```python
from build123d import *

# Parameters (mm, degrees)
SALIENTE_EXTRUIR1_DEPTH = 3


with BuildPart() as part:
    # Croquis1 → Saliente-Extruir1 (new body)
    with BuildSketch(Plane.XY):
        Polygon((-32.5, 0), (24.75, 0), (24.75, 3), (32.5, 3), (32.5, 0), (32.5, -158), (32.5, -161), (24.75, -161), (24.75, -158), (-32.5, -158), align=None)
        Polygon((-13.175, -7.03), (-25.475, -19.33), (-25.475, -7.03), align=None, mode=Mode.SUBTRACT)
        Polygon((13.175, -7.03), (25.475, -7.03), (25.475, -19.33), align=None, mode=Mode.SUBTRACT)
        Polygon((13.175, -79), (25.475, -66.7), (25.475, -91.3), align=None, mode=Mode.SUBTRACT)
        Polygon((13.175, -150.97), (25.475, -138.67), (25.475, -150.97), align=None, mode=Mode.SUBTRACT)
        Polygon((-13.175, -79), (-25.475, -66.7), (-25.475, -91.3), align=None, mode=Mode.SUBTRACT)
        Polygon((13.175, -43.015), (25.475, -55.315), (25.475, -30.715), align=None, mode=Mode.SUBTRACT)
        Polygon((-13.175, -43.015), (-25.475, -30.715), (-25.475, -55.315), align=None, mode=Mode.SUBTRACT)
        Polygon((0, -48.7075), (-12.3, -61.0075), (0, -73.3075), (12.3, -61.0075), align=None, mode=Mode.SUBTRACT)
        Polygon((0, -12.7225), (12.3, -25.0225), (0, -37.3225), (-12.3, -25.0225), align=None, mode=Mode.SUBTRACT)
        Polygon((-13.175, -150.97), (-25.475, -150.97), (-25.475, -138.67), align=None, mode=Mode.SUBTRACT)
        Polygon((-13.175, -114.985), (-25.475, -127.285), (-25.475, -102.685), align=None, mode=Mode.SUBTRACT)
        Polygon((-12.3, -132.9775), (0, -145.2775), (12.3, -132.9775), (0, -120.6775), align=None, mode=Mode.SUBTRACT)
        Polygon((13.175, -114.985), (25.475, -127.285), (25.475, -102.685), align=None, mode=Mode.SUBTRACT)
        Polygon((0, -84.6925), (12.3, -96.9925), (0, -109.2925), (-12.3, -96.9925), align=None, mode=Mode.SUBTRACT)
    extrude(amount=SALIENTE_EXTRUIR1_DEPTH)


solid = part.part
```
CAD build for the part. Positions are in the model's coordinates, mm. Round coordinates to 2 decimals unless told otherwise and drop trailing zeros. Order: outer loops, then holes, each group sorted by start corner. A loop starts at its lowest first (then second) coordinate and runs counter-clockwise, first axis right, second up.
Q1. Slice it at D-D (x = -15). Write the cut outline in (y, z) (3 decimals).
Q2. Slice it at B-B (x = 6). Write the cut outline in (y, z), and give its area (3 significant figures).
Q3. Two-plate mould, pull along Y, no slides. Class faces 1 (the flat face through (19, -7.03, 1)), 2 (the flat face through (19.41, -36.78, 1.48)), 3 (the flat face through (24.75, 1, 1)): pulls with the +Y half, pulls with the -Y half, needs draft (parallel to the pull), parting line crosses it, or undercut.
Q4. Slice it at A-A (y = -46.5). Write the cut outline in (x, z) (3 decimals), and give its area (3 significant figures).
Q5. Wall check: L1, parallel to Y at x = 14, z = 1.1 (3 decimals); L2, parallel to Y at x = -21, z = 2.4 (3 decimals); L3, parallel to X at y = -34, z = 1.35 (1 decimal). Give the ranges that are in metal, low to high.
Q6. Slice it at C-C (z = 1.4). State how many separate pieces and enclosed holes the cut face has, and give its area (3 significant figures).
Q7. Drop flat-ended pins along their axis: pin 1 (0.9 mm diameter, centred on x = 22, z = 1, fed in from +Y); pin 2 (0.9 mm diameter, centred on y = 2, z = 2, fed in from -X); pin 3 (4 mm diameter, centred on x = 3, y = -29.5, fed in from +Z). Give the stop position or say it passes through.
Results below:
1. outline: (-158, 0) - (-150.97, 0) - (-150.97, 3) - (-158, 3) - close; (-149.145, 0) - (-116.81, 0) - (-116.81, 3) - (-149.145, 3) - close; (-113.16, 0) - (-80.825, 0) - (-80.825, 3) - (-113.16, 3) - close; (-77.175, 0) - (-44.84, 0) - (-44.84, 3) - (-77.175, 3) - close; (-41.19, 0) - (-8.855, 0) - (-8.855, 3) - (-41.19, 3) - close; (-7.03, 0) - (0, 0) - (0, 3) - (-7.03, 3) - close
2. outline: (-158, 0) - (-139.28, 0) - (-139.28, 3) - (-158, 3) - close; (-126.68, 0) - (-103.29, 0) - (-103.29, 3) - (-126.68, 3) - close; (-90.69, 0) - (-67.31, 0) - (-67.31, 3) - (-90.69, 3) - close; (-54.71, 0) - (-31.32, 0) - (-31.32, 3) - (-54.71, 3) - close; (-18.72, 0) - (0, 0) - (0, 3) - (-18.72, 3) - close
2. area: 323 mm2
3. face 1: undercut
3. face 2: undercut
3. face 3: needs draft
4. outline: (-32.5, 0) - (-25.475, 0) - (-25.475, 3) - (-32.5, 3) - close; (-16.66, 0) - (16.66, 0) - (16.66, 3) - (-16.66, 3) - close; (25.475, 0) - (32.5, 0) - (32.5, 3) - (25.475, 3) - close
4. area: 142 mm2
5. L1: y = -158 to -150.97, -150.145 to -115.81, -114.16 to -79.825, -78.175 to -43.84, -42.19 to -7.855, -7.03 to 0
5. L2: y = -158 to -150.97, -143.145 to -122.81, -107.16 to -86.825, -71.175 to -50.84, -35.19 to -14.855, -7.03 to 0
5. L3: x = -32.5 to -25.5, -22.2 to -3.3, 3.3 to 22.2, 25.5 to 32.5
6. separate pieces: 1
6. enclosed holes: 14
6. area: 7,900 mm2
7. pin 1: stops at y = 0
7. pin 2: stops at x = 24.75
7. pin 3: passes through
